Here's the drawing with two shaded views (mm, measured from the low corner). I have some questions. Round coordinates to 2 decimals unless told otherwise and drop trailing zeros. Loops run counter-clockwise (first coordinate to the right, second up) from the corner with the lowest first, then second, coordinate; pieces in that order, holes last. Notation, with made-up numbers: M -26.5,-23.75 L 27.5,-23.75 A10 cw 27.5,-16.75 Z; hole C 44.5,85 d4. An arc over 180 degrees is marked long. One line per item, written item: value. Start each with the question number.
Q1. I'm going to push flat-ended pins straight in: pin 1 Ø1.6 at (x, z) = (40, 1) entering from -Y; pin 2 Ø1.5 at (x, z) = (38.5, 1) entering from +Y; pin 3 Ø1.5 at (x, z) = (31.5, 1) entering from +Y. Where does each tip first touch, or does it pass through?
Q2. Imagine slicing it at B-B (y = 12.25). Please give me the cut outline in (x, z), then the cut area to 3 significant figures.
Q3. Imagine slicing it at D-D (x = 46). Please give me the cut outline in (y, z).
Q4. Please list where these lines run through material, in increasing order: line 1 along X through (y, z) = (10.5, 0.3); line 2 along Y through (x, z) = (19.5, 1.2); line 3 along X through (y, z) = (2, 2.7).
Q5. Imagine slicing it at A-A (y = 7.75). Please give me the cut outline in (x, z), then the cut area to 3 significant figures.
Q6. Imagine slicing it at C-C (x = 54). Please give me the cut outline in (y, z), then the cut area to 3 significant figures.
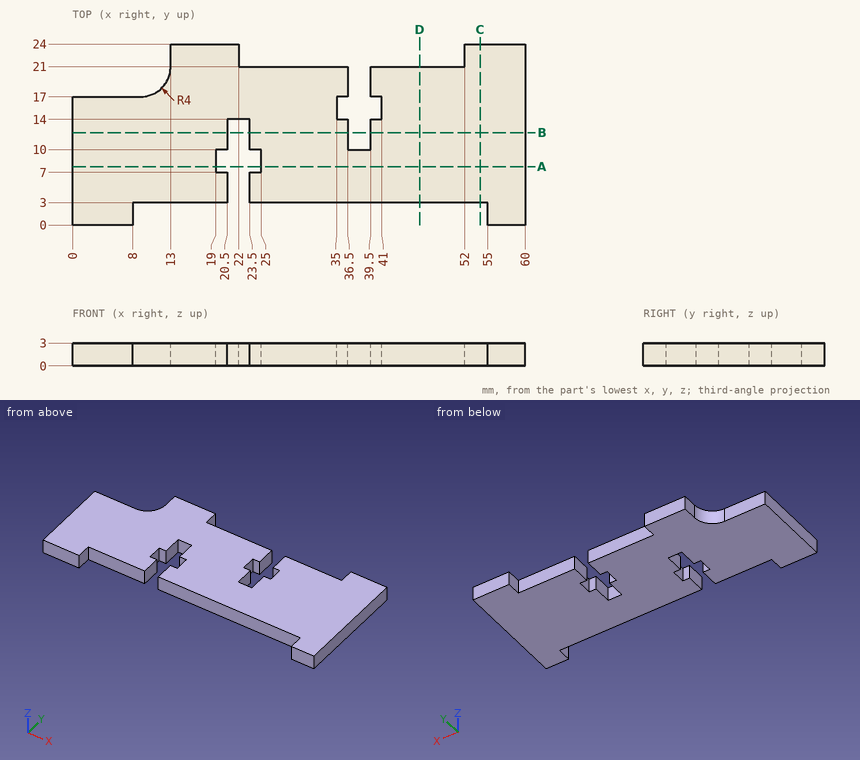
Report:
1. pin 1: stops at y = 3
1. pin 2: stops at y = 10
1. pin 3: stops at y = 21
2. outline: M 0,0 L 20.5,0 L 20.5,3 L 0,3 Z; M 23.5,0 L 36.5,0 L 36.5,3 L 23.5,3 Z; M 39.5,0 L 60,0 L 60,3 L 39.5,3 Z
2. area: 162 mm²
3. outline: M 3,0 L 21,0 L 21,3 L 3,3 Z
4. line 1: x = 0 to 20.5, 23.5 to 36.5, 39.5 to 60
4. line 2: y = 3 to 7, 10 to 24
4. line 3: x = 0 to 8, 55 to 60
5. outline: M 0,0 L 19,0 L 19,3 L 0,3 Z; M 25,0 L 60,0 L 60,3 L 25,3 Z
5. area: 162 mm²
6. outline: M 3,0 L 24,0 L 24,3 L 3,3 Z
6. area: 63.0 mm²
